The model under review builds one solid part; all positions refer to its coordinate system, in mm. A direction names the side the tool comes from. Coordinates: 2 decimals unless noted, no trailing zeros. Loops run counter-clockwise (first coordinate to the right, second up) from the corner with the lowest first, then second, coordinate; pieces in that order, holes last. Notation, with made-up numbers: M 63.25,-17.75 L 94.25,-17.75 A34 ccw 94.25,19.25 Z; hole C -32,-26 d9. An arc over 180 degrees is marked long. Use one line per item in the form item = value.
```python
from build123d import *

# Parameters (mm, degrees)
CYLINDER_R             = 1.2
CYLINDER_DEPTH         = 7.7
CYLINDER_ROLL_ANGLE    = 90
CYLINDER002_R          = 4
CYLINDER002_DEPTH      = 10
CYLINDER002_ROLL_ANGLE = 90
CYLINDER001_R          = 25
CYLINDER001_DEPTH      = 15
CYLINDER001_ROLL_ANGLE = 90
THICKNESS_T            = -3


with BuildPart() as motorshaft:
    # Cylinder → Cylinder (new body)
    with BuildSketch(Plane.XY):
        Circle(CYLINDER_R)
    extrude(amount=CYLINDER_DEPTH)


with BuildPart() as motorshaft_1:
    # Cylinder roll: moved
    add(motorshaft.part.rotate(Axis((0, 0, 0), (1, 0, 0)), CYLINDER_ROLL_ANGLE))


with BuildPart() as motorshaft_2:
    # Cylinder placement: moved
    add(motorshaft_1.part.moved(Location((0, -26.7, 0))))


with BuildPart() as shaft_holder_f:
    # Cylinder002 → Cylinder002 (new body)
    with BuildSketch(Plane.XY):
        Circle(CYLINDER002_R)
    extrude(amount=CYLINDER002_DEPTH)


with BuildPart() as shaft_holder_f_1:
    # Cylinder002 roll: moved
    add(shaft_holder_f.part.rotate(Axis((0, 0, 0), (1, 0, 0)), CYLINDER002_ROLL_ANGLE))


with BuildPart() as shaft_holder_f_2:
    # Cylinder002 placement: moved
    add(shaft_holder_f_1.part.moved(Location((0, -28, 0))))


with BuildPart() as wheel_shaft_hollow_f:
    # Cylinder001 → Cylinder001 (new body)
    with BuildSketch(Plane.XY):
        Circle(CYLINDER001_R)
    extrude(amount=CYLINDER001_DEPTH)


with BuildPart() as wheel_shaft_hollow_f_1:
    # Cylinder001 roll: moved
    add(wheel_shaft_hollow_f.part.rotate(Axis((0, 0, 0), (1, 0, 0)), CYLINDER001_ROLL_ANGLE))


with BuildPart() as wheel_shaft_hollow_f_2:
    # Cylinder001 placement: moved
    add(wheel_shaft_hollow_f_1.part.moved(Location((0, -28, 0))))

    # Thickness
    thickness_openings = [wheel_shaft_hollow_f_2.faces().sort_by_distance(p)[0] for p in [
        (0, -43, 0),
    ]]
    offset(amount=THICKNESS_T, openings=thickness_openings)

    # Fusion: union shaft_holder_f
    add(shaft_holder_f_2.part)

    # Cut: cut motorshaft
    add(motorshaft_2.part, mode=Mode.SUBTRACT)


solid = wheel_shaft_hollow_f_2.part
```
1. Add section D-D (y = -39.75). State the section outline as (x, z) points.
Response values:
outline = C 0,0 d50; hole C 0,0 d44
2. The part is to be moulded in two halves that separate along X. For faces 4 (the face through (23.846, -35.395, 7.509)), 5 (the face through (1.7, -43, -22.1)), 6 (the face through (0, -34.4, 0)), say which applies: pulls with the +X half, pulls with the -X half, needs draft (parallel to the pull), parting line crosses it, or undercut.
Response values:
face_4 = parting line crosses it
face_5 = needs draft
face_6 = undercut
3. Insertion check: P1, Ø4, axis at x = 13, y = -36, coming from the -Z side; P2, Ø4, axis at x = -0.5, z = 0, coming from the -Y side; P3, Ø1.9, axis at x = 0, z = 0, coming from the +Y side. Each pin has a flat end and moves straight along its axis. Give the tip position at first contact, or say it passes through.
Response values:
P1 = -22.45
P2 = -38
P3 = -34.4
4. Wall thickness on line 1 along Z through (x, y) = (0, -36); line 2 along Z through (x, y) = (0, -30.75); line 3 along Y through (x, z) = (0, -12.5): over which ranges is each line inside the solid? List them lowest first. Write a range as from..to.
Response values:
line_1 = -25..-22, -4..4, 22..25
line_2 = -25..-1.2, 1.2..25
line_3 = -31..-28
5. Add section B-B (y = -32). State the section outline as (x, z) points, then the cut area to 3 significant figures.
Response values:
outline = C 0,0 d50; C 0,0 d8; hole C 0,0 d44; hole C 0,0 d2.4
area = 489 mm^2
6. Add section A-A (x = 0). State the section outline as (y, z) points.
Response values:
outline = M -43,-25 L -28,-25 L -28,-1.2 L -34.4,-1.2 L -34.4,1.2 L -28,1.2 L -28,25 L -43,25 L -43,22 L -31,22 L -31,4 L -38,4 L -38,-4 L -31,-4 L -31,-22 L -43,-22 Z
7. Add section C-C (z = 0). State the section outline as (x, y) points.
Response values:
outline = M -25,-43 L -22,-43 L -22,-31 L -4,-31 L -4,-38 L 4,-38 L 4,-31 L 22,-31 L 22,-43 L 25,-43 L 25,-28 L 1.2,-28 L 1.2,-34.4 L -1.2,-34.4 L -1.2,-28 L -25,-28 Z
8. Machinability: for faces 1 (the face through (0, -28, -5)), 2 (the face through (0.65, -31.16, 1.01)), 3 (the face through (-0.867, -34.451, -3.905)), which of the approach directions +Z, -Z, +X, -X, +Y, -Y give a long, thin tool a straight path to every point of the face, cutting with its end or side? Answer none if there is none.
Response values:
face_1 = +Z, -Z, +X, -X, +Y
face_2 = +Y
face_3 = -Y
